from build123d import *

# Parameters (mm, degrees)
SKETCH2_W           = 86.5
SKETCH2_H           = 45.5
BOSS_EXTRUDE1_DEPTH = 4.5
SKETCH3_R           = 1.625
SKETCH3_R_2         = 2.38125
CUT_EXTRUDE1_DEPTH  = 5.5
SKETCH4_W           = 5.5
SKETCH4_H           = 7
CUT_EXTRUDE2_DEPTH  = 5.5
CHAMFER1_SIZE       = 0.5
SKETCH5_R           = 10
BOSS_EXTRUDE2_DEPTH = 4.5
SKETCH6_R           = 5
SKETCH6_W           = 2.5
SKETCH6_H           = 1.5
CUT_EXTRUDE3_DEPTH  = 5.5


with BuildPart() as part:
    # Sketch2 → Boss-Extrude1 (new body)
    with BuildSketch(Plane(origin=(0, 0, 0), x_dir=(1, 0, 0), z_dir=(0, 1, 0))):
        with Locations((1.75, 0)):
            Rectangle(SKETCH2_W, SKETCH2_H)
    extrude(amount=BOSS_EXTRUDE1_DEPTH)

    # Sketch3 → Cut-Extrude1 (cut, through all)
    with BuildSketch(Plane(origin=(0, 4.5, 0), x_dir=(1, 0, 0), z_dir=(0, 1, 0))):
        with Locations((-37.5, -16)):
            Circle(SKETCH3_R)
        with Locations((-37.5, 16)):
            Circle(SKETCH3_R)
        with Locations((41, 16)):
            Circle(SKETCH3_R)
        with Locations((41, -16)):
            Circle(SKETCH3_R)
        with Locations((25, 0)):
            Circle(SKETCH3_R_2)
        with Locations((-25, 0)):
            Circle(SKETCH3_R_2)
    extrude(amount=-CUT_EXTRUDE1_DEPTH, mode=Mode.SUBTRACT)

    # Sketch4 → Cut-Extrude2 (cut, through all)
    with BuildSketch(Plane(origin=(0, 4.5, 0), x_dir=(1, 0, 0), z_dir=(0, 1, 0))):
        with Locations((-19.75, 7)):
            Rectangle(SKETCH4_W, SKETCH4_H)
        with Locations((-19.75, -7)):
            Rectangle(SKETCH4_W, SKETCH4_H)
        with Locations((-19.75, 17)):
            Rectangle(SKETCH4_W, SKETCH4_H)
        with Locations((-19.75, -17)):
            Rectangle(SKETCH4_W, SKETCH4_H)
    cut_extrude2 = extrude(amount=-CUT_EXTRUDE2_DEPTH, mode=Mode.SUBTRACT)

    # Mirror1: Cut-Extrude2 across plane
    add(cut_extrude2.mirror(Plane(origin=(0, 0, 0), x_dir=(0, 0, 1), z_dir=(1, 0, 0))), mode=Mode.SUBTRACT)

    # Chamfer1
    chamfer1_edges = [part.edges().sort_by_distance(p)[0] for p in [
        (22.5, 2.25, -10.5),
        (22.5, 2.25, -3.5),
        (17, 2.25, -3.5),
        (17, 2.25, -10.5),
        (22.5, 2.25, 3.5),
        (22.5, 2.25, 10.5),
        (17, 2.25, 10.5),
        (17, 2.25, 3.5),
        (22.5, 2.25, -20.5),
        (22.5, 2.25, -13.5),
        (17, 2.25, -13.5),
        (17, 2.25, -20.5),
        (22.5, 2.25, 13.5),
        (22.5, 2.25, 20.5),
        (17, 2.25, 20.5),
        (17, 2.25, 13.5),
        (-22.5, 2.25, -3.5),
        (-22.5, 2.25, -10.5),
        (-17, 2.25, -10.5),
        (-17, 2.25, -3.5),
        (-22.5, 2.25, 10.5),
        (-22.5, 2.25, 3.5),
        (-17, 2.25, 3.5),
        (-17, 2.25, 10.5),
        (-22.5, 2.25, -13.5),
        (-22.5, 2.25, -20.5),
        (-17, 2.25, -20.5),
        (-17, 2.25, -13.5),
        (-22.5, 2.25, 20.5),
        (-22.5, 2.25, 13.5),
        (-17, 2.25, 13.5),
        (-17, 2.25, 20.5),
    ]]
    chamfer(chamfer1_edges, length=CHAMFER1_SIZE)

    # Sketch5 → Boss-Extrude2 (add)
    with BuildSketch(Plane(origin=(0, 4.5, 0), x_dir=(1, 0, 0), z_dir=(0, 1, 0))):
        with Locations((40, 0)):
            Circle(SKETCH5_R)
    extrude(amount=-BOSS_EXTRUDE2_DEPTH)

    # Sketch6 → Cut-Extrude3 (cut, through all)
    with BuildSketch(Plane(origin=(0, 4.5, 0), x_dir=(1, 0, 0), z_dir=(0, 1, 0))):
        with Locations((40, 0)):
            Circle(SKETCH6_R)
        with Locations((-40.25, -22)):
            Rectangle(SKETCH6_W, SKETCH6_H)
        with Locations((-40.25, 22)):
            Rectangle(SKETCH6_W, SKETCH6_H)
    extrude(amount=-CUT_EXTRUDE3_DEPTH, mode=Mode.SUBTRACT)


solid = part.part
For this review, take the finished solid that the model builds, in its own axes (mm). A direction names the side the tool comes from. Give positions to 0.01 mm unless a question says otherwise; leave off trailing zeros. Loops run counter-clockwise (first coordinate to the right, second up) from the corner with the lowest first, then second, coordinate; pieces in that order, holes last.
Item 1: For line 1 along Z through (x, y) = (-37.5, 1) (3 decimals); line 2 along X through (y, z) = (1.2, -16) (3 decimals); line 3 along X through (y, z) = (2.7, 0), list the stretches that pass through material, from the lowest coordinate up.
Item 2: Draft analysis for pull direction X (two halves, no side actions). For faces 1 (the flat face through (-41.5, 2, 0)), 2 (the flat face through (4, 0, 0)), 3 (the cylindrical face through (39.71, 2.28, 16.99)), state which applies: +X half, -X half, draft (parallel to the pull), parting line (faces both ways), or undercut.
Item 3: Take a section at C-C, the plane z = -19. State the section outline as (x, y) points, and give its area (3 significant figures).
Item 4: Insertion check: pin 1 (4 mm diameter, centred on x = 41, z = 16, fed in from +Y); pin 2 (1.3 mm diameter, centred on y = 2.5, z = -18.5, fed in from +X); pin 3 (0.8 mm diameter, centred on x = -40, y = 2, fed in from -Z). Each pin has a flat end and moves straight along its axis. Give the tip position at first contact, or say it passes through.
Item 5: Take a section at A-A, the plane z = 0. State the section outline as (x, y) points, and give its area (3 significant figures).
Item 6: Tool access review of faces 4 (the flat face through (20, 2, -10.5)), 5 (the flat face through (45, 2, 16)), 6 (the flat face through (-40, 2, 21.25)): name each direction out of +Z, -Z, +X, -X, +Y, -Y from which nothing blocks a thin tool from reaching the whole face with its end or side.
Item 7: Take a section at D-D, the plane z = 16. State the section outline as (x, y) points (3 decimals).
Item 8: Take a section at B-B, the plane x = -25. State the section outline as (y, z) points, and give its area (3 significant figures).
Calculated:
1. line 1: z = -22.75 to -17.625, -14.375 to 14.375, 17.625 to 22.75
1. line 2: x = -41.5 to -39.125, -35.875 to -22.5, -17 to 17, 22.5 to 39.375, 42.625 to 45
1. line 3: x = -41.5 to -27.38, -22.62 to 22.62, 27.38 to 35, 45 to 50
2. face 1: -X half
2. face 2: draft
2. face 3: undercut
3. outline: (-41.5, 0) - (-22.5, 0) - (-22.5, 4.5) - (-41.5, 4.5) - close; (-17, 0) - (17, 0) - (17, 4.5) - (-17, 4.5) - close; (22.5, 0) - (45, 0) - (45, 4.5) - (22.5, 4.5) - close
3. area: 340 mm2
4. pin 1: stops at y = 4.5
4. pin 2: stops at x = 45
4. pin 3: stops at z = -21.25
5. outline: (-41.5, 0) - (-27.38, 0) - (-27.38, 4.5) - (-41.5, 4.5) - close; (-22.62, 0) - (22.62, 0) - (22.62, 4.5) - (-22.62, 4.5) - close; (27.38, 0) - (35, 0) - (35, 4.5) - (27.38, 4.5) - close; (45, 0) - (50, 0) - (50, 4.5) - (45, 4.5) - close
5. area: 324 mm2
6. face 4: +Y, -Y
6. face 5: +Z, +X, +Y, -Y
6. face 6: +Z, -X, +Y, -Y
7. outline: (-41.5, 0) - (-39.125, 0) - (-39.125, 4.5) - (-41.5, 4.5) - close; (-35.875, 0) - (-22.5, 0) - (-22.5, 4.5) - (-35.875, 4.5) - close; (-17, 0) - (17, 0) - (17, 4.5) - (-17, 4.5) - close; (22.5, 0) - (39.375, 0) - (39.375, 4.5) - (22.5, 4.5) - close; (42.625, 0) - (45, 0) - (45, 4.5) - (42.625, 4.5) - close
8. outline: (0, -22.75) - (4.5, -22.75) - (4.5, -2.38) - (0, -2.38) - close; (0, 2.38) - (4.5, 2.38) - (4.5, 22.75) - (0, 22.75) - close
8. area: 183 mm2
